Geometry check sheet. Reference: the model listing, model coordinates, mm. A direction names the side the tool comes from. Coordinates: 2 decimals unless noted, no trailing zeros. Loops run counter-clockwise (first coordinate to the right, second up) from the corner with the lowest first, then second, coordinate; pieces in that order, holes last. Notation, with made-up numbers: (-22, 15) - (29, 15) arc R12 cw to (29, 22) - close; hole circle Ø2 at (78.5, -27.75). An arc over 180 degrees is marked (long way). Write item = value, one per line. Start each with the question number.
from build123d import *

# Parameters (mm, degrees)
SKETCH4_W            = 66.5
SKETCH4_H            = 39.6
BOSS_EXTRUDE4_DEPTH  = 2
SKETCH5_W            = 66.5
SKETCH5_H            = 39.6
SKETCH5_W_2          = 62.5
SKETCH5_H_2          = 35.6
BOSS_EXTRUDE5_DEPTH  = 4
SKETCH6_R            = 2.5
BOSS_EXTRUDE8_DEPTH  = 3
SKETCH7_R            = 0.75
CUT_EXTRUDE1_DEPTH   = 2
SKETCH9_W            = 64.5
SKETCH9_H            = 37.6
SKETCH9_W_2          = 62.5
SKETCH9_H_2          = 35.6
BOSS_EXTRUDE9_DEPTH  = 2.2
CHAMFER1_SIZE        = 0.2
CHAMFER2_SIZE        = 0.2
SKETCH11_W           = 3
SKETCH11_H           = 2
BOSS_EXTRUDE10_DEPTH = 3
FILLET1_R            = 1


with BuildPart() as part:
    # Sketch4 → Boss-Extrude4 (new body)
    with BuildSketch(Plane.XY):
        with Locations((30.75, 17.3)):
            Rectangle(SKETCH4_W, SKETCH4_H)
    extrude(amount=BOSS_EXTRUDE4_DEPTH)

    # Sketch5 → Boss-Extrude5 (add)
    with BuildSketch(Plane.XY.offset(2)):
        with Locations((30.75, 17.3)):
            Rectangle(SKETCH5_W, SKETCH5_H)
        with Locations((30.75, 17.3)):
            Rectangle(SKETCH5_W_2, SKETCH5_H_2, mode=Mode.SUBTRACT)
    extrude(amount=BOSS_EXTRUDE5_DEPTH)

    # Sketch6 → Boss-Extrude8 (add)
    with BuildSketch(Plane.XY.offset(2)):
        with Locations(Location((3.5, 6.1, 0), (0, 0, 180))):
            Circle(SKETCH6_R)
        with BuildLine():
            Line((59.5, 12.6), (62, 12.6))
            Line((62, 12.6), (62, 17.6))
            Line((62, 17.6), (59.5, 17.6))
            ThreePointArc((59.5, 17.6), (57, 15.1), (59.5, 12.6))
        make_face()
    extrude(amount=BOSS_EXTRUDE8_DEPTH)

    # Sketch7 → Cut-Extrude1 (cut)
    with BuildSketch(Plane.XY.offset(5)):
        with Locations((59.5, 15.1)):
            Circle(SKETCH7_R)
        with Locations((3.5, 6.1)):
            Circle(SKETCH7_R)
    extrude(amount=-CUT_EXTRUDE1_DEPTH, mode=Mode.SUBTRACT)

    # Sketch9 → Boss-Extrude9 (add)
    with BuildSketch(Plane.XY.offset(6)):
        with Locations((30.75, 17.3)):
            Rectangle(SKETCH9_W, SKETCH9_H)
        with Locations((30.75, 17.3)):
            Rectangle(SKETCH9_W_2, SKETCH9_H_2, mode=Mode.SUBTRACT)
    extrude(amount=BOSS_EXTRUDE9_DEPTH)

    # Chamfer1
    chamfer1_edges = [part.edges().sort_by_distance(p)[0] for p in [
        (2.75, 6.1, 5),
    ]]
    chamfer(chamfer1_edges, length=CHAMFER1_SIZE)

    # Chamfer2
    chamfer2_edges = [part.edges().sort_by_distance(p)[0] for p in [
        (58.75, 15.1, 5),
    ]]
    chamfer(chamfer2_edges, length=CHAMFER2_SIZE)

    # Sketch11 → Boss-Extrude10 (add)
    with BuildSketch(Plane.XY.offset(2)):
        with Locations((4, 34.1)):
            Rectangle(SKETCH11_W, SKETCH11_H)
        with Locations((30.75, 34.1)):
            Rectangle(SKETCH11_W, SKETCH11_H)
        with Locations((57.5, 34.1)):
            Rectangle(SKETCH11_W, SKETCH11_H)
        with Locations((30.75, 0.5)):
            Rectangle(SKETCH11_W, SKETCH11_H)
    extrude(amount=BOSS_EXTRUDE10_DEPTH)

    # Fillet1
    fillet1_edges = [part.edges().sort_by_distance(p)[0] for p in [
        (-1.5, 36.1, 7.1),
        (-2.5, 37.1, 3),
        (-1.5, -1.5, 7.1),
        (-2.5, -2.5, 3),
        (63, 36.1, 7.1),
        (63, -1.5, 7.1),
        (64, -2.5, 3),
        (64, 37.1, 3),
        (-0.5, -0.5, 5.1),
        (-0.5, 35.1, 5.1),
        (62, -0.5, 5.1),
        (62, 35.1, 5.1),
        (62, 12.6, 3.5),
        (62, 17.6, 3.5),
        (32.25, -0.5, 3.5),
        (29.25, -0.5, 3.5),
        (56, 35.1, 3.5),
        (59, 35.1, 3.5),
        (32.25, 35.1, 3.5),
        (29.25, 35.1, 3.5),
        (5.5, 35.1, 3.5),
        (2.5, 35.1, 3.5),
        (29.25, 1.5, 3.5),
        (32.25, 1.5, 3.5),
        (59, 33.1, 3.5),
        (56, 33.1, 3.5),
        (32.25, 33.1, 3.5),
        (29.25, 33.1, 3.5),
        (5.5, 33.1, 3.5),
        (2.5, 33.1, 3.5),
    ]]
    fillet(fillet1_edges, radius=FILLET1_R - 0.0001)  # a hair under: the kernel refuses the full size


solid = part.part
(1) Depth check by flat-ended pin: pin 1 (2 mm diameter, centred on x = 3.5, y = 34, fed in from +Z); pin 2 (0.7 mm diameter, centred on y = 25, z = 7, fed in from -X); pin 3 (12 mm diameter, centred on x = 42.5, y = 13.5, fed in from +Z). Enter the tip coordinate at first touch or a pass-through.
(2) Sectioned sample at A-A on x = 21. Enter the section's corners in (y, z), plus the area to 3 significant figures.
(3) Sectioned sample at D-D on z = 4. Count the separate pieces of the cut face and the enclosed holes in it, plus the area to 3 significant figures.
(4) Tool access check on faces 1 (the face through (31, 34, 5)), 2 (the face through (30.6, 35.5, 8.2)). Record the directions out of +Z, -Z, +X, -X, +Y, -Y that give a thin tool (end or side, any length) a straight path to the whole face; none if there is none.
(5) Scan lines: line 1 (Y direction, x = 3.5, z = 4.4); line 2 (X direction, y = 29, z = 4.5); line 3 (Y direction, x = 59.5, z = 4.1). Record each from-to range of solid material in increasing order.
(6) Sectioned sample at B-B on y = 6.1. Enter the section's corners in (x, z).
(7) Sectioned sample at C-C on z = 6.75. Enter the section's corners in (x, y).
(8) Draft check along Y on faces 3 (the face through (64, 17, 3)), 4 (the face through (57, 34, 5)), 5 (the face through (30, -1.5, 7)). Enter one of: pulls with the +Y half, pulls with the -Y half, needs draft (parallel to the pull), parting line crosses it, or undercut.
Working result:
q1.pin_1 = 5
q1.pin_2 = -1.5
q1.pin_3 = 2
q2.outline = (-2.5, 0) - (37.1, 0) - (37.1, 6) - (36.1, 6) - (36.1, 8.2) - (35.1, 8.2) - (35.1, 2) - (-0.5, 2) - (-0.5, 8.2) - (-1.5, 8.2) - (-1.5, 6) - (-2.5, 6) - close
q2.area = 99.6 mm2
q3.separate_pieces = 2
q3.enclosed_holes = 3
q3.area = 471 mm2
q4.face_1 = +Z
q4.face_2 = +Z, +X, -X, +Y, -Y
q5.line_1 = -2.5 to -0.5, 3.6 to 5.35, 6.85 to 8.6, 33.1 to 37.1
q5.line_2 = -2.5 to -0.5, 62 to 64
q5.line_3 = -2.5 to -0.5, 12.6 to 14.35, 15.85 to 17.6, 34.97 to 37.1
q6.outline = (-2.5, 0) - (64, 0) - (64, 6) - (63, 6) - (63, 8.2) - (62, 8.2) - (62, 2) - (6, 2) - (6, 5) - (4.45, 5) - (4.25, 4.8) - (4.25, 3) - (2.75, 3) - (2.75, 4.8) - (2.55, 5) - (1, 5) - (1, 2) - (-0.5, 2) - (-0.5, 8.2) - (-1.5, 8.2) - (-1.5, 6) - (-2.5, 6) - close
q7.outline = (-1.5, -0.5) arc R1 ccw to (-0.5, -1.5) - (62, -1.5) arc R1 ccw to (63, -0.5) - (63, 35.1) arc R1 ccw to (62, 36.1) - (-0.5, 36.1) arc R1 ccw to (-1.5, 35.1) - close; hole (-0.5, 0.5) arc R1 ccw to (0.5, -0.5) - (61, -0.5) arc R1 ccw to (62, 0.5) - (62, 34.1) arc R1 ccw to (61, 35.1) - (0.5, 35.1) arc R1 ccw to (-0.5, 34.1) - close
q8.face_3 = needs draft
q8.face_4 = undercut
q8.face_5 = pulls with the -Y half
